Can you work these out from the model? Positions are in its coordinate system, mm. Face numbers are marked on the shaded views. A direction names the side the tool comes from. Give positions to 0.01 mm unless a question says otherwise; leave off trailing zeros. Loops run counter-clockwise (first coordinate to the right, second up) from the corner with the lowest first, then second, coordinate; pieces in that order, holes last. Notation, with made-up numbers: (86.25, -39) - (138.25, -39) arc R16 ccw to (138.25, -21) - close; hole circle Ø5 at (75.25, 59.25). An arc over 180 degrees is marked (long way). Answer in a Markdown table with one row per item.
from build123d import *

# Parameters (mm, degrees)
ESBO_O1_R                = 1.4
RESSALTO_EXTRUS_O1_DEPTH = 1.4


with BuildPart() as part:
    # Esboço1 → Ressalto-extrusão1 (new body)
    with BuildSketch(Plane.XY):
        with BuildLine():
            Line((-5.101054411, 3.084372914), (-9.361488568, 2.387210962))
            ThreePointArc((-9.361488568, 2.387210962), (-9.9620658, 2.047835966), (-10.2, 1.400336379))
            Line((-10.2, 1.400336379), (-10.2, -1.400336379))
            ThreePointArc((-10.2, -1.400336379), (-9.9620658, -2.047835966), (-9.361488568, -2.387210962))
            Line((-9.361488568, -2.387210962), (-5.101054411, -3.084372914))
            ThreePointArc((-5.101054411, -3.084372914), (-4.698664301, -3.133566222), (-4.293611571, -3.15))
            Line((-4.293611571, -3.15), (7.4, -3.15))
            Line((7.4, -3.15), (7.4, -1.9))
            Line((7.4, -1.9), (10.2, -1.9))
            Line((10.2, -1.9), (10.2, -0.8))
            Line((10.2, -0.8), (9.8, 0))
            Line((9.8, 0), (10.2, 0.8))
            Line((10.2, 0.8), (10.2, 1.9))
            Line((10.2, 1.9), (7.4, 1.9))
            Line((7.4, 1.9), (7.4, 3.15))
            Line((7.4, 3.15), (-4.293611571, 3.15))
            ThreePointArc((-4.293611571, 3.15), (-4.698664301, 3.133566222), (-5.101054411, 3.084372914))
        make_face()
        with Locations((-5.5, 0)):
            Circle(ESBO_O1_R, mode=Mode.SUBTRACT)
    extrude(amount=RESSALTO_EXTRUS_O1_DEPTH)


solid = part.part
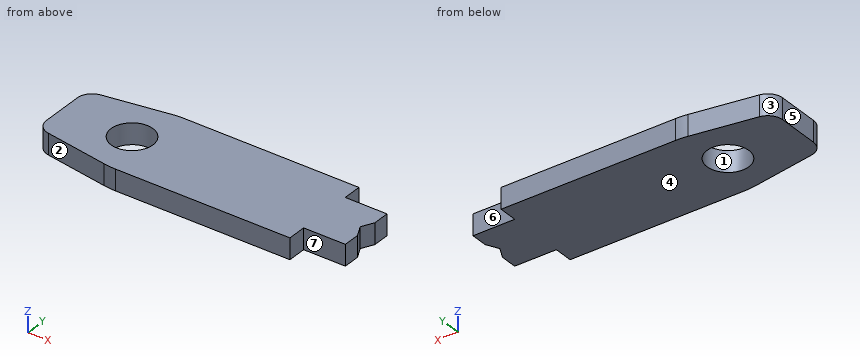
Q1. Imagine slicing it at B-B, the plane x = -5.5. Write out the boundary of the cut face in (y, z).
Checked values:
| item | result |
|---|---|
| outline | (-3.02, 0) - (-1.4, 0) - (-1.4, 1.4) - (-3.02, 1.4) - close; (1.4, 0) - (3.02, 0) - (3.02, 1.4) - (1.4, 1.4) - close |
Q2. Imagine slicing it at A-A, the plane z = 0.5. Write out the boundary of the cut face in (x, y), and give its area (3 significant figures).
Checked values:
| item | result |
|---|---|
| outline | (-10.2, -1.4) arc R1 ccw to (-9.36, -2.39) - (-5.1, -3.08) arc R5 ccw to (-4.29, -3.15) - (7.4, -3.15) - (7.4, -1.9) - (10.2, -1.9) - (10.2, -0.8) - (9.8, 0) - (10.2, 0.8) - (10.2, 1.9) - (7.4, 1.9) - (7.4, 3.15) - (-4.29, 3.15) arc R5 ccw to (-5.1, 3.08) - (-9.36, 2.39) arc R1 ccw to (-10.2, 1.4) - close; hole circle Ø2.8 at (-5.5, 0) |
| area | 110 mm² |
Q3. If we mould it in two halves opening along Y, with no side actions, what happens to the marked faces 1, 2, 3 and 4? For each: released by +Y, released by -Y, zero draft, split by the parting line, or undercut.
Checked values:
| item | result |
|---|---|
| face 1 | undercut |
| face 2 | released by -Y |
| face 3 | released by +Y |
| face 4 | zero draft |
Q4. For pin 1 (2.5 mm diameter, centred on x = -5.5, y = 0, fed in from +Z), with a flat end and sliding along its axis, tell me the tip position at first contact or that it passes through.
Checked values:
| item | result |
|---|---|
| pin 1 | passes through |
Q5. On a 3-axis mill with a long thin cutter (end or side, diameter ignored), from which of +Z, -Z, +X, -X, +Y, -Y can I reach the whole of each face in a straight line? I mean the marked faces 5, 6 and 7. Say none if no direction works.
Checked values:
| item | result |
|---|---|
| face 5 | +Z, -Z, -X, +Y, -Y |
| face 6 | +Z, -Z, +X, +Y |
| face 7 | +Z, -Z, +X, -Y |
Q6. If I drill on line 1 (Y direction, x = -5.5, z = 0.4); line 2 (X direction, y = 1.25, z = 1.1); line 3 (X direction, y = 0.25, z = 0.35) (1 decimal), over which ranges is the centre line in solid material (lowest first)? Write a range as [from, to].
Checked values:
| item | result |
|---|---|
| line 1 | y = [-3.02, -1.4], [1.4, 3.02] |
| line 2 | x = [-10.2, -6.13], [-4.87, 10.2] |
| line 3 | x = [-10.2, -6.9], [-4.1, 9.9] |
